Verification items for the finished model (mm, model axes). Face numbers are marked on the shaded views. A direction names the side the tool comes from. Give positions to 0.01 mm unless a question says otherwise; leave off trailing zeros. Order: outer loops, then holes, each group sorted by start corner. A loop starts at its lowest first (then second) coordinate and runs counter-clockwise, first axis right, second up.
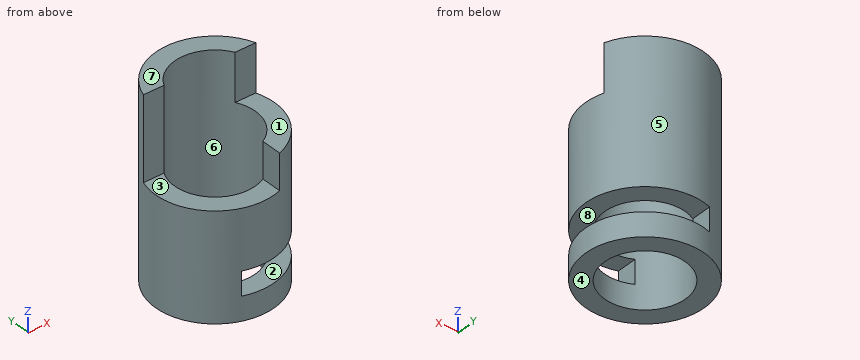
from build123d import *

# Parameters (mm, degrees)
F0_R     = 25
F1_DEPTH = 80
F2_R     = 17
F3_DEPTH = 80
F5_W     = 25
F5_H     = 35
F6_DEPTH = 33
F5_W_2   = 8
F5_H_2   = 10
F7_DEPTH = 50


with BuildPart() as f1:
    # F0 (on Top) → F1 (new body)
    with BuildSketch(Plane.XY):
        Circle(F0_R)
    extrude(amount=F1_DEPTH)

    # F2 (on face) → F3 (cut)
    with BuildSketch(Plane.XY.offset(80)):
        Circle(F2_R)
    extrude(amount=-F3_DEPTH, mode=Mode.SUBTRACT)

    # F5 (on offset) → F6 (cut)
    with BuildSketch(Plane.XZ.offset(25)):
        Polygon((0, 80), (0, 45), (8, 45), (8, 60), (25, 60), (25, 80), (8, 80), align=None)
        with Locations((-12.5, 62.5)):
            Rectangle(F5_W, F5_H)
    extrude(amount=-F6_DEPTH, mode=Mode.SUBTRACT)

    # F5 (on offset) → F7 (cut)
    with BuildSketch(Plane.XZ.offset(25)):
        with Locations((-4, 15)):
            Rectangle(F5_W_2, F5_H_2)
        with Locations((12.5, 15)):
            Rectangle(F5_W, F5_H_2)
    extrude(amount=-F7_DEPTH, mode=Mode.SUBTRACT)


solid = f1.part
(1) Scan lines: line 1 (X direction, y = 0, z = 31); line 2 (Z direction, x = 14, y = -18). Record each from-to range of solid material in increasing order.
Solved:
line 1: x = -25 to -17, 17 to 25
line 2: z = 0 to 10, 20 to 60
(2) Set-up check for the marked faces 1, 2, 3, 4 and 5: record each of +Z, -Z, +X, -X, +Y, -Y from which the full face is reachable in a straight line by a thin tool's end or side.
Solved:
face 1: +Z, +X, -X, -Y
face 2: +X, +Y, -Y
face 3: +Z, -X, -Y
face 4: -Z, +X, -X, +Y, -Y
face 5: +Z, -Z
(3) Section check B-B, the plane x = 0. Enter the section's corners in (y, z), then the cut area to 3 significant figures.
Solved:
outline: (-25, 0) - (-17, 0) - (-17, 10) - (-25, 10) - close; (-25, 20) - (-17, 20) - (-17, 45) - (-25, 45) - close; (17, 0) - (25, 0) - (25, 10) - (17, 10) - close; (17, 20) - (25, 20) - (25, 80) - (17, 80) - close
area: 840 mm2
(4) Section check A-A, the plane y = 0. Enter the section's corners in (x, z).
Solved:
outline: (-25, 0) - (-17, 0) - (-17, 45) - (-25, 45) - close; (17, 0) - (25, 0) - (25, 10) - (17, 10) - close; (17, 20) - (25, 20) - (25, 60) - (17, 60) - close
(5) Go/stop test with flat-tipped pins: pin 1 (1.5 mm diameter, centred on y = 5, z = 19, fed in from +X); pin 2 (4.5 mm diameter, centred on y = -18, z = 12.5, fed in from +X); pin 3 (4.5 mm diameter, centred on x = 20, z = 73.5, fed in from -Y). Record where each tip stops, or that it passes through.
Solved:
pin 1: stops at x = -16
pin 2: stops at x = -8
pin 3: stops at y = 8
(6) Release check for a two-part mould opening along Z. For the marked faces 6, 7 and 8 record: pulls with the +Z half, pulls with the -Z half, needs draft (parallel to the pull), parting line crosses it, or undercut.
Solved:
face 6: needs draft
face 7: pulls with the +Z half
face 8: undercut
(7) Section check D-D, the plane x = -20. Enter the section's corners in (y, z), then the cut area to 4 significant figures.
Solved:
outline: (-15, 0) - (15, 0) - (15, 80) - (8, 80) - (8, 45) - (-15, 45) - close
area: 1,595 mm2
(8) Section check C-C, the plane z = 44. Enter the section's corners in (x, y).
Solved:
outline: circle Ø50 at (0, 0); hole circle Ø34 at (0, 0)
